Geometry: see drawing. Coordinates: mm, zero at the bounding-box minimum. Coordinates: 2 decimals unless noted, no trailing zeros. Loops run counter-clockwise (first coordinate to the right, second up) from the corner with the lowest first, then second, coordinate; pieces in that order, holes last.
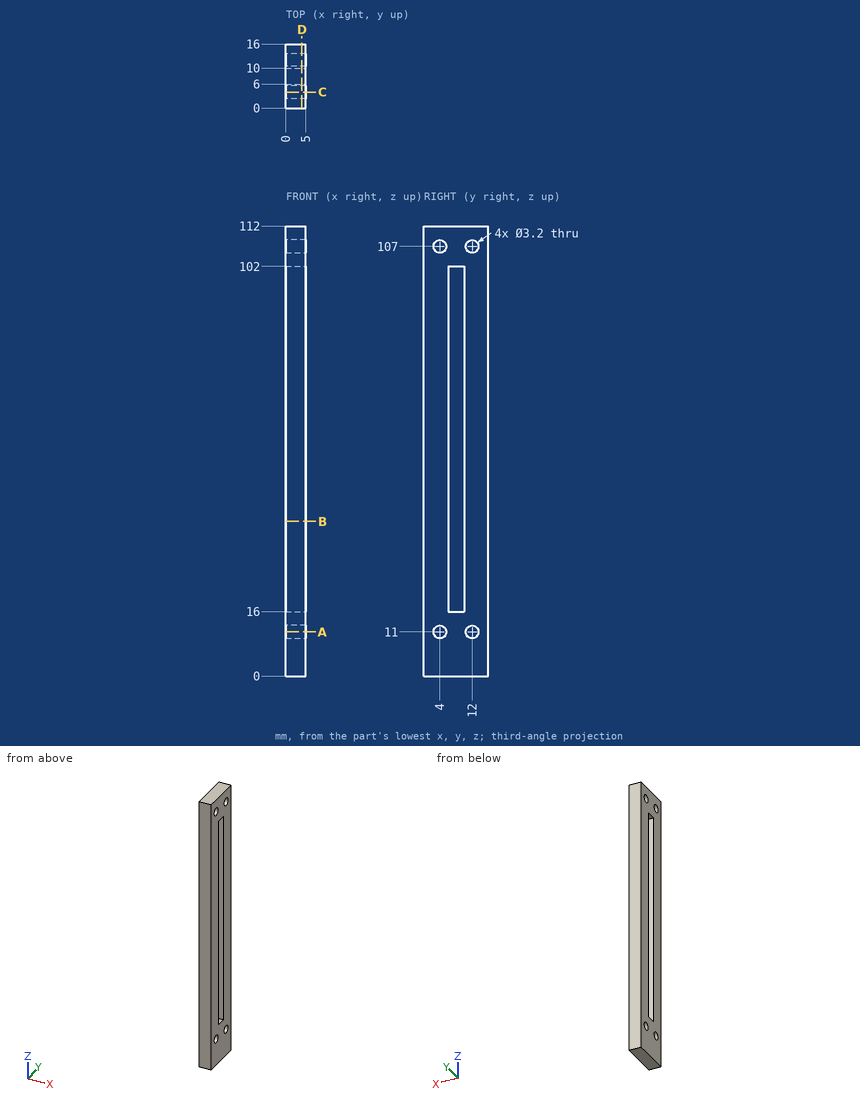
Item 1: Section query A-A (z = 11). Output: boundary loops of the cut face in (x, y), then the cut area to 3 significant figures.
Result:
outline: (0, 0) - (5, 0) - (5, 2.4) - (0, 2.4) - close; (0, 5.6) - (5, 5.6) - (5, 10.4) - (0, 10.4) - close; (0, 13.6) - (5, 13.6) - (5, 16) - (0, 16) - close
area: 48.0 mm2
Item 2: Line query: L1, parallel to Z at x = 3.65, y = 12.25; L2, parallel to Y at x = 2.85, z = 11; L3, parallel to Y at x = 3, z = 27. Output: solid intervals per line, ascending.
Result:
L1: z = 0 to 9.42, 12.58 to 105.42, 108.58 to 112
L2: y = 0 to 2.4, 5.6 to 10.4, 13.6 to 16
L3: y = 0 to 6, 10 to 16
Item 3: Section query D-D (x = 4). Output: boundary loops of the cut face in (y, z).
Result:
outline: (0, 0) - (16, 0) - (16, 112) - (0, 112) - close; hole circle Ø3.2 at (4, 11); hole circle Ø3.2 at (4, 107); hole (6, 16) - (10, 16) - (10, 102) - (6, 102) - close; hole circle Ø3.2 at (12, 11); hole circle Ø3.2 at (12, 107)
Item 4: Section query C-C (y = 4). Output: boundary loops of the cut face in (x, z), then the cut area to 3 significant figures.
Result:
outline: (0, 0) - (5, 0) - (5, 9.4) - (0, 9.4) - close; (0, 12.6) - (5, 12.6) - (5, 105.4) - (0, 105.4) - close; (0, 108.6) - (5, 108.6) - (5, 112) - (0, 112) - close
area: 528 mm2
Item 5: Contact query for flat-ended pins moving along their axis: P1, Ø3.5, axis at y = 4, z = 11, coming from the -X side; P2, Ø1.9, axis at y = 12, z = 11, coming from the +X side. Output: stop coordinate, or through.
Result:
P1: stops at x = 0
P2: passes through
Item 6: Section query B-B (z = 38.5). Output: boundary loops of the cut face in (x, y).
Result:
outline: (0, 0) - (5, 0) - (5, 6) - (0, 6) - close; (0, 10) - (5, 10) - (5, 16) - (0, 16) - close
